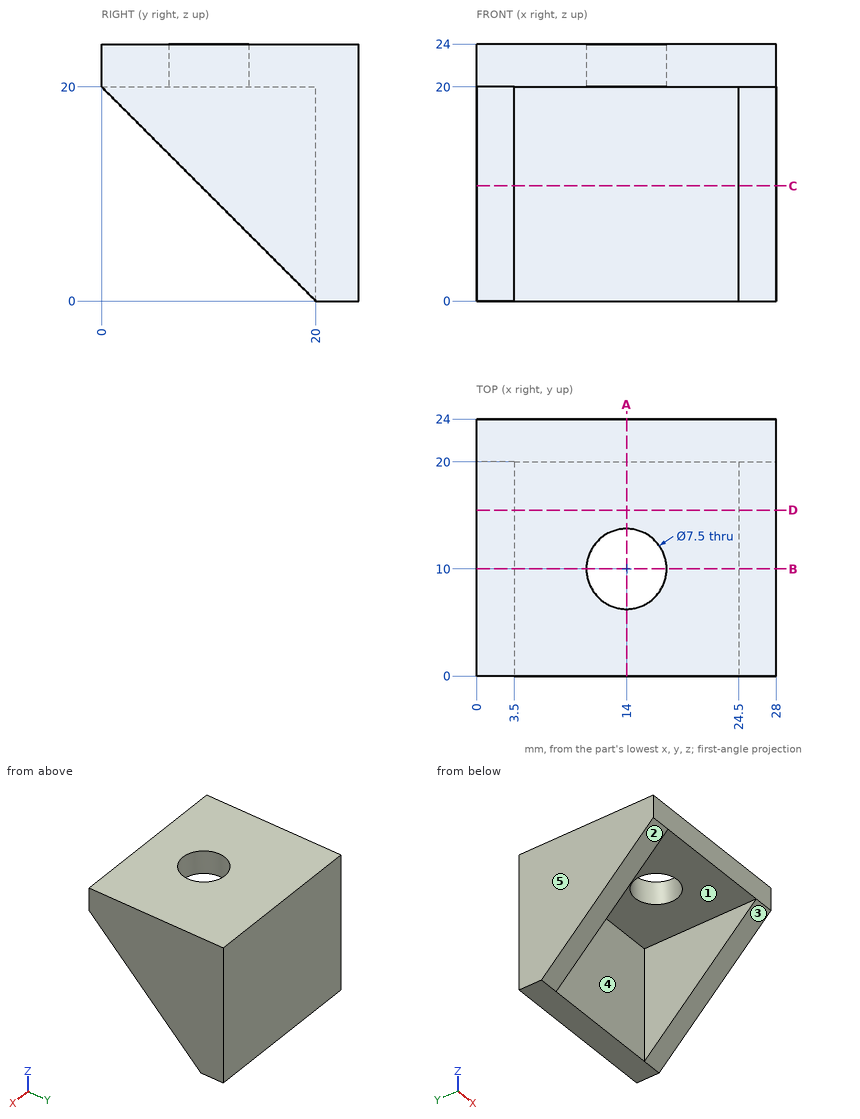
For this review, use the dimensioned drawing (mm, ordinates from the lowest corner) and the shaded views. A direction names the side the tool comes from. Coordinates: 2 decimals unless noted, no trailing zeros. Write each loop counter-clockwise with the first axis right and the second up, starting at its lowest first coordinate (ties: lowest second). Pieces come first, ordered by that corner, then holes. Notation, with made-up numbers: (44, 57) -> (53, 57) arc R13 cw to (53, 69) -> close; hole circle Ø10 at (32.5, 10). An arc over 180 degrees is marked (long way). Write each question's results on one line, items separated by ' | '. Start each with the question number.
(1) Take a section at D-D on y = 15.5. Write out the cut boundary in (x, z).
(2) Tool access review of the marked faces 1 and 2: name each direction out of +Z, -Z, +X, -X, +Y, -Y from which nothing blocks a thin tool from reaching the whole face with its end or side.
(3) For line 1 along Y through (x, z) = (14, 20.8); line 2 along Y through (x, z) = (10.25, 11.75), list the stretches that pass through material, from the lowest coordinate up. Write a range as from..to.
(4) The part is to be moulded in two halves that separate along X. For the marked faces 3, 4 and 5, say which applies: pulls with the +X half, pulls with the -X half, needs draft (parallel to the pull), parting line crosses it, or undercut.
(5) Take a section at C-C on z = 10.75. Write out the cut boundary in (x, y), and give its area (3 significant figures).
(6) Clearance check with flat-ended pins moving along their axes: P1, Ø10, axis at x = 14, y = 10, coming from the -Z side; P2, Ø3, axis at x = 22, z = 14, coming from the -Y side; P3, Ø5, axis at y = 15, z = 5, coming from the -X side. State where each tip first meets the part, or that it passes through.
(7) Take a section at A-A on x = 14. Write out the cut boundary in (y, z).
(8) Take a section at B-B on y = 10. Write out the cut boundary in (x, z), and give its area (3 significant figures).
Results found:
1) outline: (0, 4.5) -> (3.5, 4.5) -> (3.5, 20) -> (24.5, 20) -> (24.5, 4.5) -> (28, 4.5) -> (28, 24) -> (0, 24) -> close
2) face 1: -Z, -Y | face 2: -Z, +X, -X, -Y
3) line 1: y = 0..6.25, 13.75..24 | line 2: y = 20..24
4) face 3: needs draft | face 4: undercut | face 5: pulls with the -X half
5) outline: (0, 9.25) -> (3.5, 9.25) -> (3.5, 20) -> (24.5, 20) -> (24.5, 9.25) -> (28, 9.25) -> (28, 24) -> (0, 24) -> close | area: 187 mm2
6) P1: stops at z = 20 | P2: stops at y = 20 | P3: stops at x = 0
7) outline: (0, 20) -> (6.25, 20) -> (6.25, 24) -> (0, 24) -> close; (13.75, 20) -> (20, 20) -> (20, 0) -> (24, 0) -> (24, 24) -> (13.75, 24) -> close
8) outline: (0, 10) -> (3.5, 10) -> (3.5, 20) -> (10.25, 20) -> (10.25, 24) -> (0, 24) -> close; (17.75, 20) -> (24.5, 20) -> (24.5, 10) -> (28, 10) -> (28, 24) -> (17.75, 24) -> close | area: 152 mm2
